Design review of the part built by this model. Coordinates are the model's own, in mm. A direction names the side the tool comes from. Coordinates: 2 decimals unless noted, no trailing zeros. Loops run counter-clockwise (first coordinate to the right, second up) from the corner with the lowest first, then second, coordinate; pieces in that order, holes last. Notation, with made-up numbers: (24, 24) - (78, 24) arc R13 cw to (78, 47) - close; hole circle Ø7 at (47, 27.5). An arc over 180 degrees is marked (long way). Use one line per item in the form item = value. Start each with the question number.
(1) For L1, parallel to Y at x = 0, z = 1.7; L2, parallel to Y at x = 1.25, z = 2.5; L3, parallel to X at y = 20.5, z = 1.85, list the stretches that pass through material, from the lowest coordinate up.
(2) Clearance check with flat-ended pins moving along their axes: pin 1 Ø1.5 at (x, y) = (-7.5, -17) entering from +Z; pin 2 Ø5 at (y, z) = (19, 8) entering from -X; pin 3 Ø4 at (y, z) = (-1.5, 29) entering from +X; pin 4 Ø1.8 at (x, y) = (-3.5, -21.5) entering from +Z. State where each tip first meets the part, or that it passes through.
(3) The part is to be moulded in two halves that separate along Z. For faces 5 (the face through (-8, -12, 5)), 6 (the face through (-7.521, -4.534, 9.478)), 7 (the face through (-7.52, 11.21, 33.35)), 8 (the face through (3, -20.6, 1.5)), say which applies: pulls with the +Z half, pulls with the -Z half, needs draft (parallel to the pull), parting line crosses it, or undercut.
(4) Add section A-A (y = -20.5). State the section outline as (x, z) points.
(5) Add section D-D (z = 20). State the section outline as (x, y) points.
(6) Add section C-C (x = -5.5). State the section outline as (y, z) points, plus the area to 3 significant figures.
(7) Add section B-B (z = 7). State the section outline as (x, y) points, plus the area to 3 significant figures.
(8) Tool access review of faces 1 (the face through (-3, 17.5, 1)), 2 (the face through (-8, -5.5, 2)), 3 (the face through (-8, -11, 21)), 4 (the face through (-3, 20, 3)): name each direction out of +Z, -Z, +X, -X, +Y, -Y from which nothing blocks a thin tool from reaching the whole face with its end or side.
```python
from build123d import *

# Parameters (mm, degrees)
ESBO_O1_R                  = 1.65
RESSALTO_EXTRUS_O1_DEPTH   = 40
ESBO_O2_W                  = 9
ESBO_O2_H                  = 37
CORTE_EXTRUS_O1_DEPTH      = 48
ESBO_O3_R                  = 14
ESBO_O3_R_2                = 1.55
ESBO_O3_W                  = 5
ESBO_O3_H                  = 12
CORTE_EXTRUS_O2_DEPTH      = 1
CORTE_EXTRUS_O2_DEPTH_BACK = 3
FILETE1_R                  = 6


with BuildPart() as part:
    # Esboço1 → Ressalto-extrusão1 (new body)
    with BuildSketch(Plane.XY):
        with BuildLine():
            Line((0, 23.5), (-9, 23.5))
            Line((-9, 23.5), (-9, -23.5))
            Line((-9, -23.5), (0, -23.5))
            ThreePointArc((0, -23.5), (3, -20.5), (0, -17.5))
            Line((0, -17.5), (-6, -17.5))
            Line((-6, -17.5), (-6, 17.5))
            Line((-6, 17.5), (0, 17.5))
            ThreePointArc((0, 17.5), (3, 20.5), (0, 23.5))
        make_face()
        with Locations((0, 20.5)):
            Circle(ESBO_O1_R, mode=Mode.SUBTRACT)
        with Locations((0, -20.5)):
            Circle(ESBO_O1_R, mode=Mode.SUBTRACT)
    extrude(amount=RESSALTO_EXTRUS_O1_DEPTH)

    # Esboço2 → Corte-extrusão1 (cut, through all)
    with BuildSketch(Plane.XZ.offset(23.5)):
        with Locations((-1.5, 21.5)):
            Rectangle(ESBO_O2_W, ESBO_O2_H)
    extrude(amount=-CORTE_EXTRUS_O1_DEPTH, mode=Mode.SUBTRACT)

    # Esboço3 → Corte-extrusão2 (cut, two sides)
    with BuildSketch(Plane.ZY.offset(9)) as corte_extrus_o2_sk:
        with Locations((20, 7)):
            Circle(ESBO_O3_R)
        with Locations((32, 19)):
            Circle(ESBO_O3_R_2)
        with Locations((32, -5)):
            Circle(ESBO_O3_R_2)
        with Locations((8, -5)):
            Circle(ESBO_O3_R_2)
        with Locations((8, 19)):
            Circle(ESBO_O3_R_2)
        with Locations((2.5, -11.5)):
            Rectangle(ESBO_O3_W, ESBO_O3_H)
        Polygon((10, -23.5), (10, -11), (38, -11), (38, 23.5), (40, 23.5), (40, -8), (40, -23.5), align=None)
    extrude(amount=CORTE_EXTRUS_O2_DEPTH, mode=Mode.SUBTRACT)
    extrude(corte_extrus_o2_sk.sketch, amount=-CORTE_EXTRUS_O2_DEPTH_BACK, mode=Mode.SUBTRACT)

    # Filete1
    filete1_edges = [part.edges().sort_by_distance(p)[0] for p in [
        (-7.5, -11, 38),
        (-7.5, 23.5, 38),
    ]]
    fillet(filete1_edges, radius=FILETE1_R)


solid = part.part
```
Computed values:
q1.L1 = -23.5 to -22.15, -18.85 to -17.5, 17.5 to 18.85, 22.15 to 23.5
q1.L2 = -23.23 to -21.58, -19.42 to -17.77, 17.77 to 19.42, 21.58 to 23.23
q1.L3 = -9 to -1.65, 1.65 to 3
q2.pin_1 = 10
q2.pin_2 = -9
q2.pin_3 = -6
q2.pin_4 = 3
q3.face_5 = pulls with the -Z half
q3.face_6 = undercut
q3.face_7 = undercut
q3.face_8 = needs draft
q4.outline = (-9, 0) - (-1.65, 0) - (-1.65, 3) - (-6, 3) - (-6, 10) - (-9, 10) - close; (1.65, 0) - (3, 0) - (3, 3) - (1.65, 3) - close
q5.outline = (-9, -11) - (-6, -11) - (-6, -7) - (-9, -7) - close; (-9, 21) - (-6, 21) - (-6, 23.5) - (-9, 23.5) - close
q6.outline = (-23.5, 0) - (-17.5, 0) - (-17.5, 3) - (-23.5, 3) - close; (17.5, 0) - (23.5, 0) - (23.5, 3) - (17.5, 3) - close
q6.area = 36.0 mm^2
q7.outline = (-9, -23.5) - (-6, -23.5) - (-6, -6.18) - (-9, -6.18) - close; (-9, -3.82) - (-6, -3.82) - (-6, 1.8) - (-9, 1.8) - close; (-9, 12.2) - (-6, 12.2) - (-6, 17.82) - (-9, 17.82) - close; (-9, 20.18) - (-6, 20.18) - (-6, 23.5) - (-9, 23.5) - close
q7.area = 95.6 mm^2
q8.face_1 = +Z, -Z, +X
q8.face_2 = -Z, +X, -X
q8.face_3 = +Z, +X, -X, -Y
q8.face_4 = +Z, +X, +Y, -Y
